from build123d import *

# Parameters (mm, degrees)
PROFILE_R              = 1.3
PROFILE_R_2            = 1.1
PROFILE_R_3            = 2.1
EXTRUDE_289_DEPTH      = 2.8
F_2_4_START            = 2.8
F_2_4_MM_DEPTH         = 68.6
EXTRUDE_START          = 66.9
F_2_2_PROFILE_W        = 4.3
F_2_2_PROFILE_H        = 5.3
F_2_2_PROFILE_R        = 1.1
EXTRUDE_2_2_DEPTH      = 4.5
EXTRUDE_START_2        = 2.8
PROFILE_2_W            = 5
PROFILE_2_H            = 31.5
EXTRUDE_595_DEPTH      = 1.2
PROFILE_3_W            = 1.6
PROFILE_3_H            = 3.4
EXTRUDE_686_DEPTH      = 3
F_2_2_PROFILE_2_R      = 2.7
F_2_2_PROFILE_2_R_2    = 1.1
EXTRUDE_2_2_2_DEPTH    = 11.2
GNSS_START             = 2.8
GNSS_2_6_3MM_PROFILE_R = 1.3
GNSS_2_6_3MM_DEPTH     = 6
PROFILE_4_W            = 8.6
PROFILE_4_H            = 3.8
EXTRUDE_962_DEPTH      = 41.6
EXTRUDE_START_3        = 44.4
F_1_65_PROFILE_W       = 8.6
F_1_65_PROFILE_H       = 3.8
F_1_65_PROFILE_R       = 0.825
EXTRUDE_1_65_DEPTH     = 6
PROFILE_5_W            = 4.3
PROFILE_5_H            = 3.15
PROFILE_5_H_2          = 3.4
EXTRUDE_1232_DEPTH     = 31.2
EXTRUDE_START_4        = 34
F_1_65_PROFILE_2_W     = 4.3
F_1_65_PROFILE_2_H     = 3.15
F_1_65_PROFILE_2_R     = 0.825
F_1_65_PROFILE_2_H_2   = 3.4
EXTRUDE_1_65_2_DEPTH   = 6
TYPE_C_START           = 61
TYPE_C_10_11_PROFILE_W = 3.1
TYPE_C_10_11_PROFILE_H = 10
TYPE_C_10_11_DEPTH     = 11
F_7_PROFILE_R          = 3.5
CUT_EXTRUDE_7_DEPTH    = 2.5


with BuildPart() as part:
    # profile → Extrude 289 (new body)
    with BuildSketch(Plane.XY):
        Polygon((-45, -36), (45, -36), (47, -34), (47, 34), (45, 36), (-45, 36), (-47, 34), (-47, -34), align=None)
        with Locations((21.1, 3.4)):
            Circle(PROFILE_R, mode=Mode.SUBTRACT)
        with Locations((41.6, 3.4)):
            Circle(PROFILE_R, mode=Mode.SUBTRACT)
        with Locations((-32, 27.5)):
            Circle(PROFILE_R_2, mode=Mode.SUBTRACT)
        with Locations((-13, 27.5)):
            Circle(PROFILE_R_2, mode=Mode.SUBTRACT)
        with Locations((-41, -10)):
            Circle(PROFILE_R_3, mode=Mode.SUBTRACT)
        with Locations((41, -10)):
            Circle(PROFILE_R_3, mode=Mode.SUBTRACT)
        with Locations((-42, 15)):
            Circle(PROFILE_R_3, mode=Mode.SUBTRACT)
        with Locations((42, 15)):
            Circle(PROFILE_R_3, mode=Mode.SUBTRACT)
        with BuildLine():
            Line((-1.8, -33.5), (3.8, -33.5))
            ThreePointArc((3.8, -33.5), (4.5, -32.8), (3.8, -32.1))
            Line((3.8, -32.1), (-1.8, -32.1))
            ThreePointArc((-1.8, -32.1), (-2.5, -32.8), (-1.8, -33.5))
        make_face(mode=Mode.SUBTRACT)
        with BuildLine():
            Line((-1.6, 1.2), (3.6, 1.2))
            ThreePointArc((3.6, 1.2), (4.5, 2.1), (3.6, 3))
            Line((3.6, 3), (-1.6, 3))
            ThreePointArc((-1.6, 3), (-2.5, 2.1), (-1.6, 1.2))
        make_face(mode=Mode.SUBTRACT)
    extrude(amount=EXTRUDE_289_DEPTH)

    # 2.4 mm周壁 profile → 2.4 mm周壁 (add)
    with BuildSketch(Plane.XY.offset(F_2_4_START)):
        Polygon((-45, -36), (45, -36), (47, -34), (47, 34), (45, 36), (-45, 36), (-47, 34), (-47, -34), align=None)
        Polygon((-44, -33.6), (44, -33.6), (44.6, -33), (44.6, 33), (44, 33.6), (-44, 33.6), (-44.6, 33), (-44.6, -33), align=None, mode=Mode.SUBTRACT)
    extrude(amount=F_2_4_MM_DEPTH)

    # 2.2_ profile → Extrude 2.2 (add)
    # profile 1 of 4: a face of its own
    with BuildSketch(Plane.XY.offset(EXTRUDE_START)):
        with Locations((-42.05, -31.45)):
            Rectangle(F_2_2_PROFILE_W, F_2_2_PROFILE_H)
        with Locations((-42.2, -31)):
            Circle(F_2_2_PROFILE_R, mode=Mode.SUBTRACT)
    # profile 2 of 4: a face of its own
    with BuildSketch(Plane.XY.offset(EXTRUDE_START)):
        with Locations((-42.05, 31.45)):
            Rectangle(F_2_2_PROFILE_W, F_2_2_PROFILE_H)
        with Locations((-42.2, 31)):
            Circle(F_2_2_PROFILE_R, mode=Mode.SUBTRACT)
    # profile 3 of 4: a face of its own
    with BuildSketch(Plane.XY.offset(EXTRUDE_START)):
        with Locations((42.05, -31.45)):
            Rectangle(F_2_2_PROFILE_W, F_2_2_PROFILE_H)
        with Locations((42.2, -31)):
            Circle(F_2_2_PROFILE_R, mode=Mode.SUBTRACT)
    # profile 4 of 4: a face of its own
    with BuildSketch(Plane.XY.offset(EXTRUDE_START)):
        with Locations((42.05, 31.45)):
            Rectangle(F_2_2_PROFILE_W, F_2_2_PROFILE_H)
        with Locations((42.2, 31)):
            Circle(F_2_2_PROFILE_R, mode=Mode.SUBTRACT)
    extrude(amount=EXTRUDE_2_2_DEPTH)

    # profile 2 → Extrude 595 (add)
    with BuildSketch(Plane.XY.offset(EXTRUDE_START_2)):
        with Locations((-25.5, -16.05)):
            Rectangle(PROFILE_2_W, PROFILE_2_H)
        with Locations((25.5, -16.05)):
            Rectangle(PROFILE_2_W, PROFILE_2_H)
    extrude(amount=EXTRUDE_595_DEPTH)

    # profile 3 → Extrude 686 (add)
    with BuildSketch(Plane.XY.offset(EXTRUDE_START_2)):
        with Locations((-35.7, -29.7)):
            Rectangle(PROFILE_3_W, PROFILE_3_H)
        with Locations((35.7, -29.7)):
            Rectangle(PROFILE_3_W, PROFILE_3_H)
    extrude(amount=EXTRUDE_686_DEPTH)

    # 2.2 _ profile 2 → Extrude 2.2 2 (add)
    # profile 1 of 2: a face of its own
    with BuildSketch(Plane.XY.offset(EXTRUDE_START_2)):
        with Locations((-32, 27.5)):
            Circle(F_2_2_PROFILE_2_R)
        with Locations((-32, 27.5)):
            Circle(F_2_2_PROFILE_2_R_2, mode=Mode.SUBTRACT)
    # profile 2 of 2: a face of its own
    with BuildSketch(Plane.XY.offset(EXTRUDE_START_2)):
        with Locations((-13, 27.5)):
            Circle(F_2_2_PROFILE_2_R)
        with Locations((-13, 27.5)):
            Circle(F_2_2_PROFILE_2_R_2, mode=Mode.SUBTRACT)
    extrude(amount=EXTRUDE_2_2_2_DEPTH)

    # GNSS单边凸台 Ø2.6 贯穿，板内接触3mm profile → GNSS单边凸台 Ø2.6 贯穿，板内接触3mm (add)
    with BuildSketch(Plane.XY.offset(GNSS_START)):
        Polygon((18.45, 1.2), (44.2, 1.2), (44.2, 5), (38.9, 5), (38.9, 2), (23.8, 2), (23.8, 5), (18.45, 5), align=None)
        with Locations((21.1, 3.4)):
            Circle(GNSS_2_6_3MM_PROFILE_R, mode=Mode.SUBTRACT)
        with Locations((41.6, 3.4)):
            Circle(GNSS_2_6_3MM_PROFILE_R, mode=Mode.SUBTRACT)
    extrude(amount=GNSS_2_6_3MM_DEPTH)

    # profile 4 → Extrude 962 (add)
    with BuildSketch(Plane.XY.offset(EXTRUDE_START_2)):
        with Locations((40.6, -23)):
            Rectangle(PROFILE_4_W, PROFILE_4_H)
        with Locations((-40.6, -23)):
            Rectangle(PROFILE_4_W, PROFILE_4_H)
        with Locations((40.6, -0.4)):
            Rectangle(PROFILE_4_W, PROFILE_4_H)
        with Locations((-40.6, -0.4)):
            Rectangle(PROFILE_4_W, PROFILE_4_H)
    extrude(amount=EXTRUDE_962_DEPTH)

    # 1.65_ profile → Extrude 1.65 (add)
    # profile 1 of 4: a face of its own
    with BuildSketch(Plane.XY.offset(EXTRUDE_START_3)):
        with Locations((40.6, -23)):
            Rectangle(F_1_65_PROFILE_W, F_1_65_PROFILE_H)
        with Locations((38.4, -23)):
            Circle(F_1_65_PROFILE_R, mode=Mode.SUBTRACT)
    # profile 2 of 4: a face of its own
    with BuildSketch(Plane.XY.offset(EXTRUDE_START_3)):
        with Locations((-40.6, -23)):
            Rectangle(F_1_65_PROFILE_W, F_1_65_PROFILE_H)
        with Locations((-38.4, -23)):
            Circle(F_1_65_PROFILE_R, mode=Mode.SUBTRACT)
    # profile 3 of 4: a face of its own
    with BuildSketch(Plane.XY.offset(EXTRUDE_START_3)):
        with Locations((40.6, -0.4)):
            Rectangle(F_1_65_PROFILE_W, F_1_65_PROFILE_H)
        with Locations((38.4, -0.4)):
            Circle(F_1_65_PROFILE_R, mode=Mode.SUBTRACT)
    # profile 4 of 4: a face of its own
    with BuildSketch(Plane.XY.offset(EXTRUDE_START_3)):
        with Locations((-40.6, -0.4)):
            Rectangle(F_1_65_PROFILE_W, F_1_65_PROFILE_H)
        with Locations((-38.4, -0.4)):
            Circle(F_1_65_PROFILE_R, mode=Mode.SUBTRACT)
    extrude(amount=EXTRUDE_1_65_DEPTH)

    # profile 5 → Extrude 1232 (add)
    with BuildSketch(Plane.XY.offset(EXTRUDE_START_2)):
        with Locations((-39.5, 3.025)):
            Rectangle(PROFILE_5_W, PROFILE_5_H)
        with Locations((-39.5, 32.3)):
            Rectangle(PROFILE_5_W, PROFILE_5_H_2)
        with Locations((15, 3.025)):
            Rectangle(PROFILE_5_W, PROFILE_5_H)
        with Locations((15, 32.3)):
            Rectangle(PROFILE_5_W, PROFILE_5_H_2)
    extrude(amount=EXTRUDE_1232_DEPTH)

    # 1.65_ profile 2 → Extrude 1.65 2 (add)
    # profile 1 of 4: a face of its own
    with BuildSketch(Plane.XY.offset(EXTRUDE_START_4)):
        with Locations((-39.5, 3.025)):
            Rectangle(F_1_65_PROFILE_2_W, F_1_65_PROFILE_2_H)
        with Locations((-39.5, 3.2)):
            Circle(F_1_65_PROFILE_2_R, mode=Mode.SUBTRACT)
    # profile 2 of 4: a face of its own
    with BuildSketch(Plane.XY.offset(EXTRUDE_START_4)):
        with Locations((-39.5, 32.3)):
            Rectangle(F_1_65_PROFILE_2_W, F_1_65_PROFILE_2_H_2)
        with Locations((-39.5, 32.2)):
            Circle(F_1_65_PROFILE_2_R, mode=Mode.SUBTRACT)
    # profile 3 of 4: a face of its own
    with BuildSketch(Plane.XY.offset(EXTRUDE_START_4)):
        with Locations((15, 3.025)):
            Rectangle(F_1_65_PROFILE_2_W, F_1_65_PROFILE_2_H)
        with Locations((15, 3.2)):
            Circle(F_1_65_PROFILE_2_R, mode=Mode.SUBTRACT)
    # profile 4 of 4: a face of its own
    with BuildSketch(Plane.XY.offset(EXTRUDE_START_4)):
        with Locations((15, 32.3)):
            Rectangle(F_1_65_PROFILE_2_W, F_1_65_PROFILE_2_H_2)
        with Locations((15, 32.2)):
            Circle(F_1_65_PROFILE_2_R, mode=Mode.SUBTRACT)
    extrude(amount=EXTRUDE_1_65_2_DEPTH)

    # Type-C 暂定10×11开口 profile → Type-C 暂定10×11开口 (cut)
    with BuildSketch(Plane.XY.offset(TYPE_C_START)):
        with Locations((-45.75, -9)):
            Rectangle(TYPE_C_10_11_PROFILE_W, TYPE_C_10_11_PROFILE_H)
    extrude(amount=-TYPE_C_10_11_DEPTH, mode=Mode.SUBTRACT)

    # 反面天线连接位置 Ø7预留孔 profile → 反面天线连接位置 Ø7预留孔 (cut)
    with BuildSketch(Plane.XZ.offset(36)):
        with Locations(Location((-14, 49.7, 0), (0, 0, 270))):
            Circle(F_7_PROFILE_R)
    extrude(amount=-CUT_EXTRUDE_7_DEPTH, mode=Mode.SUBTRACT)


solid = part.part
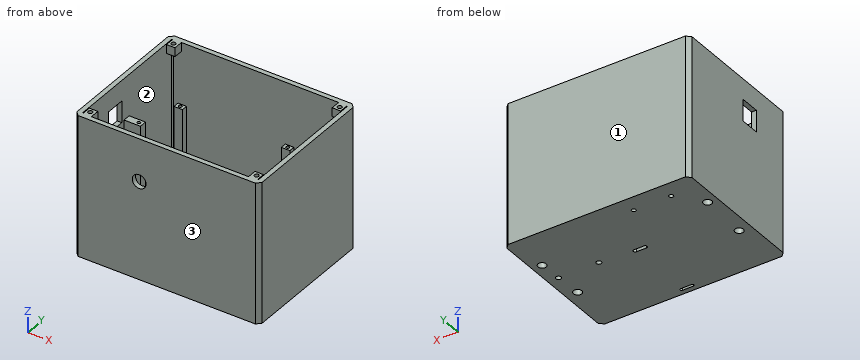
Can you work these out from the model? Positions are in its coordinate system, mm. Face numbers are marked on the shaded views. Round coordinates to 2 decimals unless told otherwise and drop trailing zeros. Loops run counter-clockwise (first coordinate to the right, second up) from the corner with the lowest first, then second, coordinate; pieces in that order, holes last. Notation, with made-up numbers: (43.25, -12.5) - (61.25, -12.5) arc R29 ccw to (61.25, 25.5) - close; hole circle Ø10 at (48.25, 25). An arc over 180 degrees is marked (long way). Answer in a Markdown table with one row per item. Add a question column.
Q1. We'd pull the mould along Y, two halves only. Please class the marked faces 1, 2 and 3: pulls with the +Y half, pulls with the -Y half, needs draft (parallel to the pull), parting line crosses it, or undercut.
Q2. I want a section at A-A on y = -19. List the corners of the cut face in (x, z) for me, and give its area (3 significant figures).
Q3. I want a section at C-C on z = 11. Count the separate pieces of the cut face and the enclosed holes in it, and give its area (3 significant figures).
Q4. For pin 1 Ø6.5 at (x, y) = (41, -10) entering from +Z; pin 2 Ø3 at (x, y) = (41, -1) entering from +Z; pin 3 Ø1.5 at (x, y) = (4.5, 21.5) entering from -Z, each with a flat end and sliding along its axis, tell me the tip position at first contact or that it passes through.
Q5. I need wall thicknesses on L1, parallel to X at y = 32.2, z = 38.1 (3 decimals); L2, parallel to X at y = 4, z = 25; L3, parallel to Y at x = 14.5, z = 23.5. Which ranges of each line are inside material? Lowest first, please.
Q6. I want a section at B-B on z = 65. List the corners of the cut face in (x, y) for me.
A:
| question | item | result |
|---|---|---|
| 1 | face 1 | pulls with the +Y half |
| 1 | face 2 | undercut |
| 1 | face 3 | pulls with the -Y half |
| 2 | outline | (-47, 0) - (47, 0) - (47, 71.4) - (44.6, 71.4) - (44.6, 2.8) - (28, 2.8) - (28, 4) - (23, 4) - (23, 2.8) - (-23, 2.8) - (-23, 4) - (-28, 4) - (-28, 2.8) - (-44.6, 2.8) - (-44.6, 71.4) - (-47, 71.4) - close |
| 2 | area | 604 mm^2 |
| 3 | separate pieces | 4 |
| 3 | enclosed holes | 3 |
| 3 | area | 984 mm^2 |
| 4 | pin 1 | z = 2.8 |
| 4 | pin 2 | z = 50.4 |
| 4 | pin 3 | z = 0 |
| 5 | L1 | -47 to -44.6, -41.65 to -40.325, -38.675 to -37.35, 12.85 to 14.175, 15.825 to 17.15, 44.6 to 47 |
| 5 | L2 | -47 to -44.6, -41.65 to -37.35, 12.85 to 17.15, 44.6 to 47 |
| 5 | L3 | -36 to -33.6, 1.45 to 4.6, 30.6 to 36 |
| 6 | outline | (-47, -34) - (-45, -36) - (45, -36) - (47, -34) - (47, 34) - (45, 36) - (-45, 36) - (-47, 34) - close; hole (-44.6, -33) - (-44, -33.6) - (44, -33.6) - (44.6, -33) - (44.6, 33) - (44, 33.6) - (-44, 33.6) - (-44.6, 33) - close |
